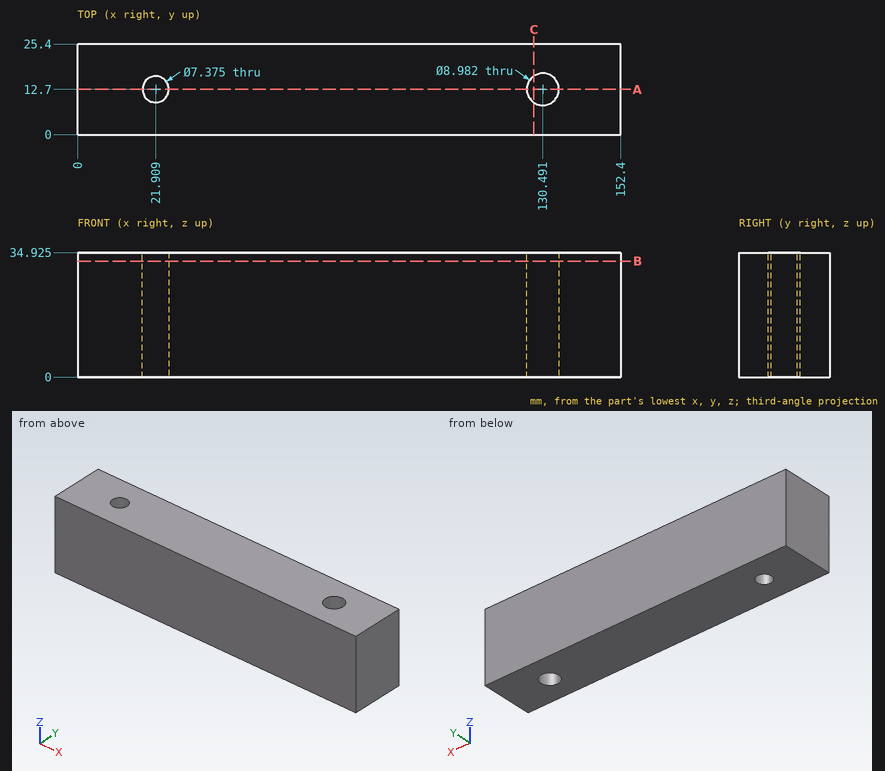
Geometry check sheet. Reference: drawing and pictorial views, mm from the part's lowest x, y, z. Round coordinates to 2 decimals unless told otherwise and drop trailing zeros. Order: outer loops, then holes, each group sorted by start corner. A loop starts at its lowest first (then second) coordinate and runs counter-clockwise, first axis right, second up. Notation, with made-up numbers: M -22.75,75 L 33.25,75 A19 ccw 33.25,100 Z; hole C 23.25,51 d5. An arc over 180 degrees is marked long. Answer in a Markdown table with one row per item.
(1) Scan lines: probe 1 along X at (y, z) = (12, 26.5) (1 decimal); probe 2 along X at (y, z) = (14.25, 19) (1 decimal); probe 3 along Y at (x, z) = (19.5, 14). Record each from-to range of solid material in increasing order. Write a range as from..to.
Responses:
| item | result |
|---|---|
| probe 1 | x = 0..18.3, 25.5..126.1, 134.9..152.4 |
| probe 2 | x = 0..18.6, 25.3..126.3, 134.7..152.4 |
| probe 3 | y = 0..9.91, 15.49..25.4 |
(2) Sectioned sample at A-A, the plane y = 12.7. Record the cut outline in (x, z) (1 decimal), and give its area (3 significant figures).
Responses:
| item | result |
|---|---|
| outline | M 0,0 L 18.2,0 L 18.2,34.9 L 0,34.9 Z; M 25.6,0 L 126,0 L 126,34.9 L 25.6,34.9 Z; M 135,0 L 152.4,0 L 152.4,34.9 L 135,34.9 Z |
| area | 4,750 mm² |
(3) Sectioned sample at C-C, the plane x = 128. Record the cut outline in (y, z) (1 decimal), and give its area (3 significant figures).
Responses:
| item | result |
|---|---|
| outline | M 0,0 L 9,0 L 9,34.9 L 0,34.9 Z; M 16.4,0 L 25.4,0 L 25.4,34.9 L 16.4,34.9 Z |
| area | 626 mm² |
(4) Sectioned sample at B-B, the plane z = 32.5. Record the cut outline in (x, y) (1 decimal).
Responses:
| item | result |
|---|---|
| outline | M 0,0 L 152.4,0 L 152.4,25.4 L 0,25.4 Z; hole C 21.9,12.7 d7.4; hole C 130.5,12.7 d9 |
(5) Go/stop test with a flat-tipped pin: P1, Ø1.5, axis at x = 133, z = 29.5, coming from the -Y side. Record where the tip stops, or that it passes through.
Responses:
| item | result |
|---|---|
| P1 | stops at y = 0 |
